from build123d import *

# Parameters (mm, degrees)
SKETCH1_W         = 8
SKETCH1_H         = 80
SKETCH1_R         = 2
MAIN_DEPTH        = 10
FIXHOLE_REACH     = 82
SKETCH3_R         = 1.25
ROLLINGHOLE_DEPTH = 9


with BuildPart() as part:
    # Sketch1 → Main (new body, symmetric)
    with BuildSketch(Plane.XY):
        with Locations((0, 30)):
            Rectangle(SKETCH1_W, SKETCH1_H)
        Circle(SKETCH1_R, mode=Mode.SUBTRACT)
    extrude(amount=MAIN_DEPTH, both=True)

    # Sketch3 → FixHole (cut, up to next)
    with BuildSketch(Plane(origin=(0, -10, 0), x_dir=(-1, 0, 0), z_dir=(0, -1, 0)), mode=Mode.PRIVATE) as fixhole_sk1:
        Circle(SKETCH3_R)
    fixhole_tool1 = extrude(fixhole_sk1.sketch, amount=-FIXHOLE_REACH, mode=Mode.PRIVATE) & part.part
    add(fixhole_tool1.solids().sort_by_distance((0, -10, 0))[0], mode=Mode.SUBTRACT)

    # Sketch4 → RollingHole (cut, through all)
    with BuildSketch(Plane.ZY.offset(4)):
        with BuildLine():
            Line((-5.2, 10), (-5.2, 60))
            ThreePointArc((-5.2, 60), (0, 65.2), (5.2, 60))
            Line((5.2, 60), (5.2, 10))
            ThreePointArc((5.2, 10), (0, 4.8), (-5.2, 10))
        make_face()
    extrude(amount=-ROLLINGHOLE_DEPTH, mode=Mode.SUBTRACT)


solid = part.part
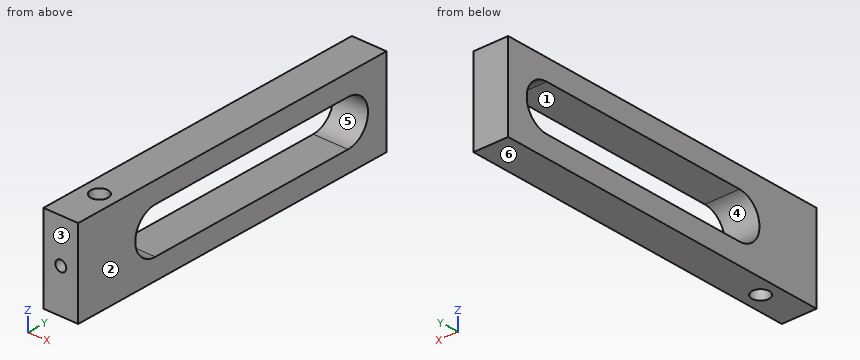
CAD build for the part. Positions are in the model's coordinates, mm. Face numbers are marked on the shaded views. A direction names the side the tool comes from. Coordinates: 2 decimals unless noted, no trailing zeros. Order: outer loops, then holes, each group sorted by start corner. A loop starts at its lowest first (then second) coordinate and runs counter-clockwise, first axis right, second up. Notation, with made-up numbers: (80, -30.75) -> (136, -30.75) arc R30 cw to (136, -0.75) -> close; hole circle Ø11 at (34.5, 8). An arc over 180 degrees is marked (long way). Answer in a Markdown table with one row per item.
1) Drill centre lines: line 1 (X direction, y = -4.25, z = 0); line 2 (Z direction, x = -3.5, y = 58); line 3 (Y direction, x = 0, z = -3.25). Where is each one in solid material? Low to high.
Check values:
| item | result |
|---|---|
| line 1 | -4 to -1.25, 1.25 to 4 |
| line 2 | -10 to -5.2, 5.2 to 10 |
| line 3 | -10 to -2, 2 to 5.94, 64.06 to 70 |
2) Band-saw the part on C-C (y = 46.5). List the corners of the cut face in (x, z).
Check values:
| item | result |
|---|---|
| outline | (-4, -10) -> (4, -10) -> (4, -5.2) -> (-4, -5.2) -> close; (-4, 5.2) -> (4, 5.2) -> (4, 10) -> (-4, 10) -> close |
3) Band-saw the part on A-A (x = 0). List the corners of the cut face in (y, z).
Check values:
| item | result |
|---|---|
| outline | (-10, -10) -> (-2, -10) -> (-2, -1.25) -> (-10, -1.25) -> close; (-10, 1.25) -> (-2, 1.25) -> (-2, 10) -> (-10, 10) -> close; (2, -10) -> (70, -10) -> (70, 10) -> (2, 10) -> close; hole (10, -5.2) -> (60, -5.2) arc R5.2 ccw to (60, 5.2) -> (10, 5.2) arc R5.2 ccw to start |
4) Which spindle directions (+Z, -Z, +X, -X, +Y, -Y) get a long thin tool onto all of the face, cutting with end or side? Do the marked faces 1 and 2. Say none if no direction does.
Check values:
| item | result |
|---|---|
| face 1 | +X, -X |
| face 2 | +Z, -Z, +X, +Y, -Y |
5) Band-saw the part on B-B (z = 0). List the corners of the cut face in (x, y), and give its area (3 significant figures).
Check values:
| item | result |
|---|---|
| outline | (-4, -10) -> (-1.25, -10) -> (-1.25, -1.56) arc R2 cw (long way) to (1.25, -1.56) -> (1.25, -10) -> (4, -10) -> (4, 4.8) -> (-4, 4.8) -> close; (-4, 65.2) -> (4, 65.2) -> (4, 70) -> (-4, 70) -> close |
| area | 124 mm2 |
6) Mould opens along Y. For the marked faces 3, 4, 5 and 6 say: pulls with the +Y half, pulls with the -Y half, needs draft (parallel to the pull), parting line crosses it, or undercut.
Check values:
| item | result |
|---|---|
| face 3 | pulls with the -Y half |
| face 4 | undercut |
| face 5 | undercut |
| face 6 | needs draft |
7) Band-saw the part on D-D (z = -4.25). List the corners of the cut face in (x, y), and give its area (3 significant figures).
Check values:
| item | result |
|---|---|
| outline | (-4, -10) -> (4, -10) -> (4, 7) -> (-4, 7) -> close; (-4, 63) -> (4, 63) -> (4, 70) -> (-4, 70) -> close; hole circle Ø4 at (0, 0) |
| area | 179 mm2 |
